Part model, mm, in its own coordinate system. A direction names the side the tool comes from. Round coordinates to 2 decimals unless told otherwise and drop trailing zeros. Write each loop counter-clockwise with the first axis right and the second up, starting at its lowest first coordinate (ties: lowest second). Pieces come first, ordered by that corner, then holes.
```python
from build123d import *


with BuildPart() as part:
    # 草图1 → 旋转1 (revolve)
    with BuildSketch(Plane.XY, mode=Mode.PRIVATE) as revolve_1_sk:
        Polygon((0, 0), (0, 14.5), (-6, 14.5), (-6, 18.5), (0, 18.5), (0, 29), (6, 29), (6, 0), align=None)
    revolve(revolve_1_sk.sketch.rotate(Axis((0, 0, 0), (-1, 0, 0)), 90), axis=Axis((0, 0, 0), (-1, 0, 0)))

    # 草图2 → 切除-旋转1 (revolve, cut)
    with BuildSketch(Plane.XY, mode=Mode.PRIVATE) as cut_revolve_1_sk:
        Polygon((0, 0), (0, 8.5), (2, 8.5), (2, 12.5), (4, 12.5), (4, 8.5), (6, 8.5), (6, 0), align=None)
    revolve(cut_revolve_1_sk.sketch.rotate(Axis((0, 0, 0), (-1, 0, 0)), 90), axis=Axis((0, 0, 0), (-1, 0, 0)), mode=Mode.SUBTRACT)


solid = part.part
```
Q1. Cut at C-C on z = -10. Write the cut outline in (x, y).
Values follow:
outline: (-6, -15.56) - (0, -15.56) - (0, -27.22) - (6, -27.22) - (6, 27.22) - (0, 27.22) - (0, 15.56) - (-6, 15.56) - (-6, 10.5) - (0, 10.5) - (0, -10.5) - (-6, -10.5) - close; hole (2, -7.5) - (4, -7.5) - (4, 7.5) - (2, 7.5) - close
Q2. Wall check: L1, parallel to Y at x = 5.15, z = 0; L2, parallel to Y at x = 3.5, z = 0; L3, parallel to X at y = -15, z = -21. Give the ranges that are in metal, low to high.
Values follow:
L1: y = -29 to -8.5, 8.5 to 29
L2: y = -29 to -12.5, 12.5 to 29
L3: x = 0 to 6
Q3. Cut at D-D on x = -3.25. Write the cut outline in (y, z), plus the area to 3 significant figures.
Values follow:
outline: circle Ø37 at (0, 0); hole circle Ø29 at (0, 0)
area: 415 mm2
Q4. Which spindle directions (+Z, -Z, +X, -X, +Y, -Y) get a long thin tool onto all of the face, cutting with end or side? Do faces 4 (the flat face through (-6, 10, -11)), 5 (the flat face through (4, 8.2, 3)), 6 (the cylindrical face through (-3.042, 12.864, -6.691)). Say none if no direction does.
Values follow:
face 4: +Z, -Z, -X, +Y, -Y
face 5: none
face 6: -X
Q5. Mould opens along Y. For faces 1 (the cylindrical face through (-2.96, 16.41, -8.54)), 2 (the cylindrical face through (5.014, -8.428, 1.107)), 3 (the flat face through (6, -7, -6)) say: +Y half, -Y half, draft (parallel to the pull), parting line (faces both ways), or undercut.
Values follow:
face 1: parting line
face 2: undercut
face 3: draft
Q6. Drop flat-ended pins along their axis: pin 1 (4 mm diameter, centred on x = -0.5, z = -3.5, fed in from -Y); pin 2 (4 mm diameter, centred on x = 1.5, y = -17.5, fed in from +Z); pin 3 (1 mm diameter, centred on x = 2, y = -18.5, fed in from -Z); pin 4 (10 mm diameter, centred on y = 0, z = 0, fed in from +X). Give the stop position or say it passes through.
Values follow:
pin 1: stops at y = -28.96
pin 2: stops at z = 24.51
pin 3: stops at z = -22.74
pin 4: passes through
Q7. Cut at A-A on z = 0. Write the cut outline in (x, y), plus the area to 3 significant figures.
Values follow:
outline: (-6, -18.5) - (0, -18.5) - (0, -29) - (6, -29) - (6, -8.5) - (4, -8.5) - (4, -12.5) - (2, -12.5) - (2, -8.5) - (0, -8.5) - (0, -14.5) - (-6, -14.5) - close; (-6, 14.5) - (0, 14.5) - (0, 8.5) - (2, 8.5) - (2, 12.5) - (4, 12.5) - (4, 8.5) - (6, 8.5) - (6, 29) - (0, 29) - (0, 18.5) - (-6, 18.5) - close
area: 278 mm2
